from build123d import *

# Parameters (mm, degrees)
SKETCH1_W                = 2.5
SKETCH1_H                = 30
SKETCH2_R                = 6
BOSS_EXTRUDE1_DEPTH      = 1
SKETCH3_R                = 4.4
BOSS_EXTRUDE2_DEPTH      = 1.5
CHAMFER1_SIZE            = 1.8
BOSS_EXTRUDE3_DEPTH      = 3
BOSS_EXTRUDE3_DEPTH_BACK = 1.5
CHAMFER2_SIZE            = 0.2
CHAMFER2_EDGE_2_SIZE     = 0.2
CHAMFER2_EDGE_3_SIZE     = 0.2
CHAMFER2_EDGE_4_SIZE     = 0.2
CHAMFER2_EDGE_5_SIZE     = 0.2
CHAMFER2_EDGE_6_SIZE     = 0.2


with BuildPart() as part:
    # Sketch1 → Revolve1 (revolve)
    with BuildSketch(Plane(origin=(0, 0, 0), x_dir=(1, 0, 0), z_dir=(0, 1, 0)), mode=Mode.PRIVATE) as revolve1_sk:
        with Locations((1.25, 15)):
            Rectangle(SKETCH1_W, SKETCH1_H)
    revolve(revolve1_sk.sketch.rotate(Axis((0, 0, -30), (0, 0, 1)), 180), axis=Axis((0, 0, -30), (0, 0, 1)))

    # Sketch2 → Boss-Extrude1 (add)
    with BuildSketch(Plane.XY):
        Circle(SKETCH2_R)
    extrude(amount=BOSS_EXTRUDE1_DEPTH)

    # Sketch3 → Boss-Extrude2 (add)
    with BuildSketch(Plane.XY.offset(1)):
        Circle(SKETCH3_R)
    extrude(amount=BOSS_EXTRUDE2_DEPTH)

    # Chamfer1
    # the kernel refuses this chamfer: 1.8 mm, written as the material it adds along each edge
    with BuildSketch(Plane(origin=(0, 0, 1), x_dir=(1, 0, 0), z_dir=(0, -1, 0))) as chamfer1_piece_1_section:
        Polygon((4.4 + CHAMFER1_SIZE, 0), (4.4, CHAMFER1_SIZE), (4.4, 0), align=None)
    chamfer1_piece_1 = revolve(axis=Axis((0, 0, 1), (0, 0, 1)), mode=Mode.PRIVATE)
    chamfer1_piece_1 = chamfer1_piece_1 & Plane(origin=(0, 0, 1.82351745), x_dir=(1, 0, 0), z_dir=(0, 0, -1)) * Cylinder(6, 25, mode=Mode.PRIVATE)
    chamfer1_piece_1 = split(chamfer1_piece_1, bisect_by=Plane(origin=(-5.32351745, 0, 2.5), z_dir=(0, 0, -1)), keep=Keep.TOP, mode=Mode.PRIVATE)
    add(chamfer1_piece_1)

    # Sketch4 → Boss-Extrude3 (add, two sides: drawn at the far end of the back side and taken through both)
    with BuildSketch(Plane.XY.offset(2.5).offset(-BOSS_EXTRUDE3_DEPTH_BACK)):
        Polygon((-2.309401077, 4), (-4.618802154, 0), (-2.309401077, -4), (2.309401077, -4), (4.618802154, 0), (2.309401077, 4), align=None)
    extrude(amount=BOSS_EXTRUDE3_DEPTH + BOSS_EXTRUDE3_DEPTH_BACK)

    # Chamfer2
    chamfer2_edges = [part.edges().sort_by_distance(p)[0] for p in [
        (-2.309401077, 4, 4),
    ]]
    chamfer(chamfer2_edges, length=CHAMFER2_SIZE)

    # Chamfer2 edge 2
    chamfer2_edge_2_edges = [part.edges().sort_by_distance(p)[0] for p in [
        (2.309401077, 4, 4),
    ]]
    chamfer(chamfer2_edge_2_edges, length=CHAMFER2_EDGE_2_SIZE)

    # Chamfer2 edge 3
    chamfer2_edge_3_edges = [part.edges().sort_by_distance(p)[0] for p in [
        (4.618802154, 0, 4),
    ]]
    chamfer(chamfer2_edge_3_edges, length=CHAMFER2_EDGE_3_SIZE)

    # Chamfer2 edge 4
    chamfer2_edge_4_edges = [part.edges().sort_by_distance(p)[0] for p in [
        (2.309401077, -4, 4),
    ]]
    chamfer(chamfer2_edge_4_edges, length=CHAMFER2_EDGE_4_SIZE)

    # Chamfer2 edge 5
    chamfer2_edge_5_edges = [part.edges().sort_by_distance(p)[0] for p in [
        (-2.309401077, -4, 4),
    ]]
    chamfer(chamfer2_edge_5_edges, length=CHAMFER2_EDGE_5_SIZE)

    # Chamfer2 edge 6
    chamfer2_edge_6_edges = [part.edges().sort_by_distance(p)[0] for p in [
        (-4.618802154, 0, 4),
    ]]
    chamfer(chamfer2_edge_6_edges, length=CHAMFER2_EDGE_6_SIZE)


solid = part.part
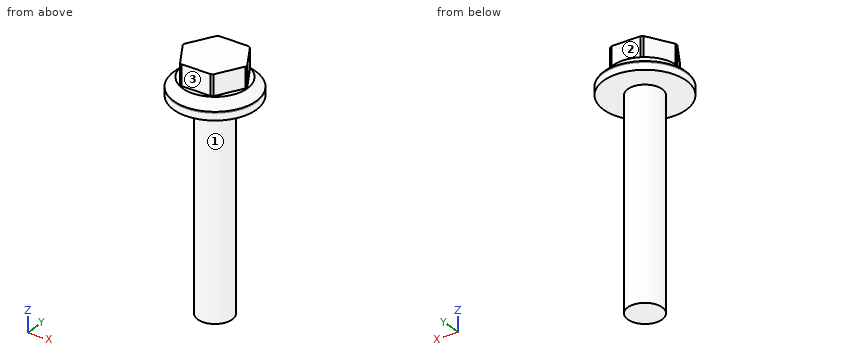
Model file for the job. Use its own axes, mm. Face numbers are marked on the shaded views. A direction names the side the tool comes from. Coordinates: 2 decimals unless noted, no trailing zeros. Loops run counter-clockwise (first coordinate to the right, second up) from the corner with the lowest first, then second, coordinate; pieces in that order, holes last. Notation, with made-up numbers: (-3.75, 56.25) -> (8.25, 56.25) arc R16 ccw to (8.25, 60.25) -> close; hole circle Ø5 at (77.25, -33.5). An arc over 180 degrees is marked (long way). Use one line per item in the form item = value. Start each with the question number.
(1) Probe probe 1 along Z at (x, y) = (-0.5, 2.5); probe 2 along Z at (x, y) = (3.25, -2.75); probe 3 along X at (y, z) = (-0.5, -2.5). List the from-to ranges inside material, lowest first. Write a range as from..to.
(2) Flat gauge pins, fed straight in: pin 1 (2 mm diameter, centred on y = 4.5, z = -7, fed in from -X); pin 2 (2 mm diameter, centred on y = -1, z = -15, fed in from -X); pin 3 (2.5 mm diameter, centred on x = 1, z = 4.5, fed in from -Y); pin 4 (4 mm diameter, centred on x = 4, z = -23.5, fed in from +Y). Where does each tip first touch, or does it go through?
(3) Tool access for the marked faces 1, 2 and 3: list every direction of +Z, -Z, +X, -X, +Y, -Y with a clear straight run to the whole face (end or side of a thin tool).
(4) Cut at B-B on z = -23. Give the cut face in (x, y).
(5) Cut at A-A on x = 0. Give the cut face in (y, z).
Values:
q1.probe_1 = 0..5.5
q1.probe_2 = 0..2.5
q1.probe_3 = -2.45..2.45
q2.pin_1 = through
q2.pin_2 = -2.5
q2.pin_3 = -4
q2.pin_4 = 1.5
q3.face_1 = -Z
q3.face_2 = +Z, +X, -X, +Y
q3.face_3 = +Z, +X, -X, -Y
q4.outline = circle Ø5 at (0, 0)
q5.outline = (-6, 0) -> (-2.5, 0) -> (-2.5, -30) -> (2.5, -30) -> (2.5, 0) -> (6, 0) -> (6, 1.2) -> (4.7, 2.5) -> (4, 2.5) -> (4, 5.5) -> (-4, 5.5) -> (-4, 2.5) -> (-4.7, 2.5) -> (-6, 1.2) -> close
